from build123d import *

# Parameters (mm, degrees)
SKETCH1_R                = 30
BOSS_EXTRUDE1_DEPTH      = 27
SKETCH3_R                = 20
CUT_EXTRUDE1_DEPTH       = 4
CUT_EXTRUDE2_START       = -4
SKETCH4_R                = 20
CUT_EXTRUDE2_DEPTH       = 4
BOSS_EXTRUDE2_DEPTH      = 10
BOSS_EXTRUDE2_DEPTH_BACK = 30
SKETCH5_R                = 2.5


with BuildPart() as part:
    # Sketch1 → Boss-Extrude1 (new body)
    with BuildSketch(Plane.XY):
        Circle(SKETCH1_R)
    extrude(amount=BOSS_EXTRUDE1_DEPTH)

    # Sketch3 → Cut-Extrude1 (cut)
    with BuildSketch(Plane.XY.offset(27)):
        Circle(SKETCH3_R)
    extrude(amount=-CUT_EXTRUDE1_DEPTH, mode=Mode.SUBTRACT)

    # Sketch4 → Cut-Extrude2 (cut)
    with BuildSketch(Plane(origin=(0, 0, 0), x_dir=(-1, 0, 0), z_dir=(0, 0, -1)).offset(CUT_EXTRUDE2_START)):
        with Locations(Location((0, 0, 0), (0, 0, 180))):
            Circle(SKETCH4_R)
    extrude(amount=CUT_EXTRUDE2_DEPTH, mode=Mode.SUBTRACT)

    # Sketch5 → Boss-Extrude2 (add, two sides: drawn at the far end of the back side and taken through both)
    with BuildSketch(Plane.XY.offset(23).offset(-BOSS_EXTRUDE2_DEPTH_BACK)):
        Circle(SKETCH5_R)
    extrude(amount=BOSS_EXTRUDE2_DEPTH + BOSS_EXTRUDE2_DEPTH_BACK)


solid = part.part
Verification items for the finished model (mm, model axes). A direction names the side the tool comes from. Give positions to 0.01 mm unless a question says otherwise; leave off trailing zeros. Loops run counter-clockwise (first coordinate to the right, second up) from the corner with the lowest first, then second, coordinate; pieces in that order, holes last. Notation, with made-up numbers: (1, -26.5) - (46, -26.5) arc R20 cw to (46, -14.5) - close; hole circle Ø7 at (58.5, 86). An arc over 180 degrees is marked (long way). Write each question's results on one line, items separated by ' | '.
1) Tool access check on faces 4 (the cylindrical face through (-19.98, -0.88, 2.03)), 5 (the flat face through (0, 0, 33)), 6 (the flat face through (4, 0, 23)). Record the directions out of +Z, -Z, +X, -X, +Y, -Y that give a thin tool (end or side, any length) a straight path to the whole face; none if there is none.
Solution:
face 4: -Z | face 5: +Z, +X, -X, +Y, -Y | face 6: +Z
2) Sectioned sample at C-C on z = -2.5. Record the boundary of the cut face in (x, y), plus the area to 3 significant figures.
Solution:
outline: circle Ø5 at (0, 0) | area: 19.6 mm2
3) Mould release check, pull along X, two halves, no side actions. Record for faces 1 (the flat face through (6, -20, 27)), 2 (the cylindrical face through (-29.97, 1.32, 13.31)), 3 (the cylindrical face through (-4.336, -19.524, 25.028)): pulls with the +X half, pulls with the -X half, needs draft (parallel to the pull), parting line crosses it, or undercut.
Solution:
face 1: needs draft | face 2: parting line crosses it | face 3: undercut
4) Material ranges on L1, parallel to Y at x = 0, z = 24; L2, parallel to Z at x = -17, y = -3; L3, parallel to Z at x = -26, y = -8.5, recorded low to high. Write a range as from..to.
Solution:
L1: -30..-20, -2.5..2.5, 20..30 | L2: 4..23 | L3: 0..27
5) Depth check by flat-ended pin: P1, Ø6, axis at y = -7.5, z = 28, coming from the +X side; P2, Ø4, axis at y = 6, z = -1, coming from the -X side; P3, Ø8, axis at y = 23.5, z = 21.5, coming from the -X side; P4, Ø1.5, axis at y = 5.5, z = -2, coming from the +X side. Enter the tip coordinate at first touch or a pass-through.
Solution:
P1: x = 29.63 | P2: x = -29.69 | P3: x = -22.8 | P4: through
6) Sectioned sample at A-A on x = 0. Record the boundary of the cut face in (y, z), plus the area to 4 significant figures.
Solution:
outline: (-30, 0) - (-20, 0) - (-20, 4) - (-2.5, 4) - (-2.5, -7) - (2.5, -7) - (2.5, 4) - (20, 4) - (20, 0) - (30, 0) - (30, 27) - (20, 27) - (20, 23) - (2.5, 23) - (2.5, 33) - (-2.5, 33) - (-2.5, 23) - (-20, 23) - (-20, 27) - (-30, 27) - close | area: 1,405 mm2
7) Sectioned sample at D-D on x = 13. Record the boundary of the cut face in (y, z), plus the area to 3 significant figures.
Solution:
outline: (-27.04, 0) - (-15.2, 0) - (-15.2, 4) - (15.2, 4) - (15.2, 0) - (27.04, 0) - (27.04, 27) - (15.2, 27) - (15.2, 23) - (-15.2, 23) - (-15.2, 27) - (-27.04, 27) - close | area: 1,220 mm2
